Geometry: final body of the model. Coordinates: model frame, mm. A direction names the side the tool comes from. Give positions to 0.01 mm unless a question says otherwise; leave off trailing zeros. Loops run counter-clockwise (first coordinate to the right, second up) from the corner with the lowest first, then second, coordinate; pieces in that order, holes last. Notation, with made-up numbers: (68.25, 44) -> (99.25, 44) arc R17 ccw to (99.25, 54) -> close; hole circle Ø10 at (32.5, 12.25). An arc over 180 degrees is marked (long way). One line per item, written item: value. Start each with the question number.
from build123d import *

# Parameters (mm, degrees)
EXTRUDE_1_DEPTH     = 15
SKETCH_2_R          = 2.5
CUT_EXTRUDE_1_DEPTH = 31.805843601
SKETCH_3_R          = 3
CUT_EXTRUDE_2_DEPTH = 40.462007045


with BuildPart() as part:
    # 草图1 → 凸台-拉伸1 (new body)
    with BuildSketch(Plane.XY):
        Polygon((-20, 0), (20, 0), (20, -6), (7.5, -6), (7.5, -24), (-7.5, -24), (-7.5, -6), (-20, -6), align=None)
    extrude(amount=EXTRUDE_1_DEPTH)

    # 草图2 → 切除-拉伸1 (cut, through all)
    with BuildSketch(Plane.XZ.offset(6)):
        with Locations(Location((15, 7.5, 0), (0, 0, 270))):
            Circle(SKETCH_2_R)
    cut_extrude_1 = extrude(amount=-CUT_EXTRUDE_1_DEPTH, mode=Mode.SUBTRACT)

    # 镜向1: 切除-拉伸1 across plane
    add(cut_extrude_1.mirror(Plane(origin=(0, 0, 0), x_dir=(0, 0, 1), z_dir=(1, 0, 0))), mode=Mode.SUBTRACT)

    # 草图3 → 切除-拉伸2 (cut, through all)
    with BuildSketch(Plane(origin=(7.5, 0, 0), x_dir=(0, 0, -1), z_dir=(1, 0, 0))):
        with Locations(Location((-7.5, -19, 0), (0, 0, 90))):
            Circle(SKETCH_3_R)
    extrude(amount=-CUT_EXTRUDE_2_DEPTH, mode=Mode.SUBTRACT)


solid = part.part
Item 1: Access query for faces 1 (the face through (-7.5, -15, 7)), 2 (the face through (0, -9, 15)), 3 (the face through (12, -6, 7)). Directions: +Z, -Z, +X, -X, +Y, -Y. A direction counts if a zero-diameter tool reaches every point of the face in a straight line with its end or side. Return the directions, or none.
Item 2: Section C-C, the plane x = 15. Output: boundary loops of the cut face in (y, z), then the cut area to 3 significant figures.
Item 3: Section A-A, the plane y = -19. Output: boundary loops of the cut face in (x, z).
Item 4: Ray query, line 1 along X through (y, z) = (-2.15, 7.5); line 2 along Z through (x, y) = (-15, -4); line 3 along Z through (x, y) = (-3.75, -19). Return the intervals inside material, ascending. Write a range as [from, to].
Item 5: Pin query (flat end, axial travel): pin 1 (6 mm diameter, centred on x = 14.5, z = 6, fed in from -Y); pin 2 (2 mm diameter, centred on x = 9, y = -8, fed in from +Z); pin 3 (4 mm diameter, centred on y = -13.5, z = 2.5, fed in from -X); pin 4 (8 mm diameter, centred on y = -20.5, z = 11.5, fed in from +X). Return the tip coordinate at first contact, or that it passes through.
Item 6: Mould query, pull axis Y, two halves, no side actions, for faces 4 (the face through (0.1, -22, 7.6)), 5 (the face through (-12, -6, 7)), 6 (the face through (-12.56, -3.04, 8.04)), 7 (the face through (0, 0, 7)). Classes: pulls with the +Y half, pulls with the -Y half, needs draft (parallel to the pull), parting line crosses it, or undercut.
Item 7: Section B-B, the plane z = 7.5. Output: boundary loops of the cut face in (x, y).
Item 8: Section D-D, the plane z = 2.25. Output: boundary loops of the cut face in (x, y).
Geometry check:
1. face 1: +Z, -Z, -X, -Y
1. face 2: +Z, +X, -X, +Y, -Y
1. face 3: +Z, -Z, +X, -Y
2. outline: (-6, 0) -> (0, 0) -> (0, 5) -> (-6, 5) -> close; (-6, 10) -> (0, 10) -> (0, 15) -> (-6, 15) -> close
2. area: 60.0 mm2
3. outline: (-7.5, 0) -> (7.5, 0) -> (7.5, 4.5) -> (-7.5, 4.5) -> close; (-7.5, 10.5) -> (7.5, 10.5) -> (7.5, 15) -> (-7.5, 15) -> close
4. line 1: x = [-20, -17.5], [-12.5, 12.5], [17.5, 20]
4. line 2: z = [0, 5], [10, 15]
4. line 3: z = [0, 4.5], [10.5, 15]
5. pin 1: stops at y = -6
5. pin 2: passes through
5. pin 3: stops at x = -7.5
5. pin 4: stops at x = 7.5
6. face 4: undercut
6. face 5: pulls with the -Y half
6. face 6: needs draft
6. face 7: pulls with the +Y half
7. outline: (-20, -6) -> (-17.5, -6) -> (-17.5, 0) -> (-20, 0) -> close; (-12.5, -6) -> (-7.5, -6) -> (-7.5, -16) -> (7.5, -16) -> (7.5, -6) -> (12.5, -6) -> (12.5, 0) -> (-12.5, 0) -> close; (-7.5, -24) -> (7.5, -24) -> (7.5, -22) -> (-7.5, -22) -> close; (17.5, -6) -> (20, -6) -> (20, 0) -> (17.5, 0) -> close
8. outline: (-20, -6) -> (-7.5, -6) -> (-7.5, -24) -> (7.5, -24) -> (7.5, -6) -> (20, -6) -> (20, 0) -> (-20, 0) -> close
